Design review of the part built by this model. Coordinates are the model's own, in mm. A direction names the side the tool comes from. Coordinates: 2 decimals unless noted, no trailing zeros. Write each loop counter-clockwise with the first axis right and the second up, starting at its lowest first coordinate (ties: lowest second). Pieces come first, ordered by that corner, then holes. Notation, with made-up numbers: (47.5, 38) - (51.5, 38) arc R11 cw to (51.5, 57) - close; hole circle Ø2 at (-22, 27). An arc over 180 degrees is marked (long way). Answer as a JSON object with one key per item and string values.
```python
from build123d import *

# Parameters (mm, degrees)
SKICA1_W                 = 55.6
SKICA1_H                 = 55.6
SKICA1_R                 = 2.4
P_IDAT_VYSUNUT_M1_DEPTH  = 1.9
SKICA2_W                 = 55.6
SKICA2_H                 = 55.6
P_IDAT_VYSUNUT_M2_DEPTH  = 0.8
SKICA3_R                 = 2.35
P_IDAT_VYSUNUT_M3_DEPTH  = 1.6
SKICA12_W                = 1
SKICA12_H                = 40
P_IDAT_VYSUNUT_M5_DEPTH  = 6
SKICA13_W                = 1
SKICA13_H                = 30
P_IDAT_VYSUNUT_M6_DEPTH  = 4
SKICA14_W                = 2
SKICA14_H                = 8
ODEBRAT_VYSUNUT_M6_DEPTH = 54
SKICA17_W                = 5.5
SKICA17_H                = 42
SKICA17_W_2              = 42
SKICA17_H_2              = 5.5
ODEBRAT_VYSUNUT_M7_DEPTH = 1.9


with BuildPart() as part:
    # Skica1 → Přidat vysunutím1 (new body)
    with BuildSketch(Plane.XY):
        Rectangle(SKICA1_W, SKICA1_H)
        with Locations((-23.9, 23.9)):
            Circle(SKICA1_R, mode=Mode.SUBTRACT)
        with Locations((23.9, 23.9)):
            Circle(SKICA1_R, mode=Mode.SUBTRACT)
        with Locations((-23.9, -23.9)):
            Circle(SKICA1_R, mode=Mode.SUBTRACT)
        with Locations((23.9, -23.9)):
            Circle(SKICA1_R, mode=Mode.SUBTRACT)
    extrude(amount=P_IDAT_VYSUNUT_M1_DEPTH)

    # Skica2 → Přidat vysunutím2 (add)
    with BuildSketch(Plane.XY.offset(1.9)):
        Rectangle(SKICA2_W, SKICA2_H)
    extrude(amount=P_IDAT_VYSUNUT_M2_DEPTH)

    # Skica3 → Přidat vysunutím3 (add)
    with BuildSketch(Plane.XY.offset(2.7)):
        with Locations((-23.9, 23.9)):
            Circle(SKICA3_R)
        with Locations((23.9, 23.9)):
            Circle(SKICA3_R)
        with Locations((-23.9, -23.9)):
            Circle(SKICA3_R)
        with Locations((23.9, -23.9)):
            Circle(SKICA3_R)
    extrude(amount=P_IDAT_VYSUNUT_M3_DEPTH)

    # Skica12 → Přidat vysunutím5 (add)
    with BuildSketch(Plane.XY.offset(2.7)):
        with Locations((-7.3, 0.5)):
            Rectangle(SKICA12_W, SKICA12_H)
        with Locations((11.7, 0)):
            Rectangle(SKICA12_W, SKICA12_H)
    extrude(amount=P_IDAT_VYSUNUT_M5_DEPTH)

    # Skica13 → Přidat vysunutím6 (add)
    with BuildSketch(Plane.XY.offset(2.7)):
        with Locations((-25.8, 1.319838769)):
            Rectangle(SKICA13_W, SKICA13_H)
        with Locations((24.7, 1.319838769)):
            Rectangle(SKICA13_W, SKICA13_H)
    extrude(amount=P_IDAT_VYSUNUT_M6_DEPTH)

    # Skica14 → Odebrat vysunutím6 (cut)
    with BuildSketch(Plane.ZY.offset(26.3)):
        with Locations((3.7, 10.319838769)):
            Rectangle(SKICA14_W, SKICA14_H)
        with Locations((3.7, -7.680161231)):
            Rectangle(SKICA14_W, SKICA14_H)
    extrude(amount=-ODEBRAT_VYSUNUT_M6_DEPTH, mode=Mode.SUBTRACT)

    # Skica17 → Odebrat vysunutím7 (cut)
    with BuildSketch(Plane(origin=(0, 0, 0), x_dir=(-1, 0, 0), z_dir=(0, 0, -1))):
        with Locations((-23.75, 0)):
            Rectangle(SKICA17_W, SKICA17_H)
        with Locations((0, 23.75)):
            Rectangle(SKICA17_W_2, SKICA17_H_2)
        Rectangle(SKICA17_W_2, SKICA17_H)
        with Locations((23.75, 0)):
            Rectangle(SKICA17_W, SKICA17_H)
        with Locations((0, -23.75)):
            Rectangle(SKICA17_W_2, SKICA17_H_2)
    extrude(amount=-ODEBRAT_VYSUNUT_M7_DEPTH, mode=Mode.SUBTRACT)


solid = part.part
```
(1) Take a section at C-C, the plane z = 5.5. Write out the cut boundary in (x, y), and give its area (3 significant figures).
Solved:
{"outline": "(-26.3, -13.68) - (-25.3, -13.68) - (-25.3, 16.32) - (-26.3, 16.32) - close; (-7.8, -19.5) - (-6.8, -19.5) - (-6.8, 20.5) - (-7.8, 20.5) - close; (11.2, -20) - (12.2, -20) - (12.2, 20) - (11.2, 20) - close; (24.2, -13.68) - (25.2, -13.68) - (25.2, 16.32) - (24.2, 16.32) - close", "area": "140 mm^2"}
(2) Take a section at D-D, the plane y = -17. Write out the cut boundary in (x, z).
Solved:
{"outline": "(-27.8, 0) - (-26.5, 0) - (-26.5, 1.9) - (26.5, 1.9) - (26.5, 0) - (27.8, 0) - (27.8, 2.7) - (12.2, 2.7) - (12.2, 8.7) - (11.2, 8.7) - (11.2, 2.7) - (-6.8, 2.7) - (-6.8, 8.7) - (-7.8, 8.7) - (-7.8, 2.7) - (-27.8, 2.7) - close"}
(3) Take a section at A-A, the plane y = 13. Write out the cut boundary in (x, z), and give its area (3 significant figures).
Solved:
{"outline": "(-27.8, 0) - (-26.5, 0) - (-26.5, 1.9) - (26.5, 1.9) - (26.5, 0) - (27.8, 0) - (27.8, 2.7) - (-27.8, 2.7) - close; (-26.3, 4.7) - (-25.3, 4.7) - (-25.3, 6.7) - (-26.3, 6.7) - close; (-7.8, 4.7) - (-6.8, 4.7) - (-6.8, 8.7) - (-7.8, 8.7) - close; (11.2, 4.7) - (12.2, 4.7) - (12.2, 8.7) - (11.2, 8.7) - close; (24.2, 4.7) - (25.2, 4.7) - (25.2, 6.7) - (24.2, 6.7) - close", "area": "61.4 mm^2"}
(4) Take a section at B-B, the plane z = 1. Write out the cut boundary in (x, y).
Solved:
{"outline": "(-27.8, -27.8) - (27.8, -27.8) - (27.8, 27.8) - (-27.8, 27.8) - close; hole (-26.5, -21) - (-21, -21) - (-21, -26.5) - (21, -26.5) - (21, -21) - (26.5, -21) - (26.5, 21) - (21, 21) - (21, 26.5) - (-21, 26.5) - (-21, 21) - (-26.5, 21) - close; hole circle Ø4.8 at (-23.9, -23.9); hole circle Ø4.8 at (-23.9, 23.9); hole circle Ø4.8 at (23.9, -23.9); hole circle Ø4.8 at (23.9, 23.9)"}
(5) For pin 1 (1.1 mm diameter, centred on x = 24.5, y = -8.5, fed in from -Z); pin 2 (2 mm diameter, centred on y = -14, z = 7.5, fed in from -X); pin 3 (0.8 mm diameter, centred on x = 25, y = 6.5, fed in from +Z), all flat-tipped, find the tip position at first contact; note any pin that passes through.
Solved:
{"pin 1": "stops at z = 1.9", "pin 2": "stops at x = -26.3", "pin 3": "stops at z = 6.7"}
(6) Tool access review of faces 3 (the face through (12.2, 0, 6)), 4 (the face through (24, -24, 4.3)), 5 (the face through (21, -24, 1)): name each direction out of +Z, -Z, +X, -X, +Y, -Y from which nothing blocks a thin tool from reaching the whole face with its end or side.
Solved:
{"face 3": "+Z, +Y, -Y", "face 4": "+Z, +X, -X, -Y", "face 5": "-Z"}
(7) To check wall thickness, follow line 1 (X direction, y = -1.5, z = 2.75); line 2 (Y direction, x = -23.9, z = 1.55); line 3 (Y direction, x = -7.5, z = 1). State the ranges of each line that lie inside material, in increasing order. Write a range as from..to.
Solved:
{"line 1": "x = -26.3..-25.3, -7.8..-6.8, 11.2..12.2, 24.2..25.2", "line 2": "y = -27.8..-26.3, -21.5..-21, 21..21.5, 26.3..27.8", "line 3": "y = -27.8..-26.5, 26.5..27.8"}
(8) The part is to be moulded in two halves that separate along Y. For faces 1 (the face through (27.8, 0, 1)), 2 (the face through (23.38, 21.557, 0.937)), say which applies: pulls with the +Y half, pulls with the -Y half, needs draft (parallel to the pull), parting line crosses it, or undercut.
Solved:
{"face 1": "needs draft", "face 2": "undercut"}
